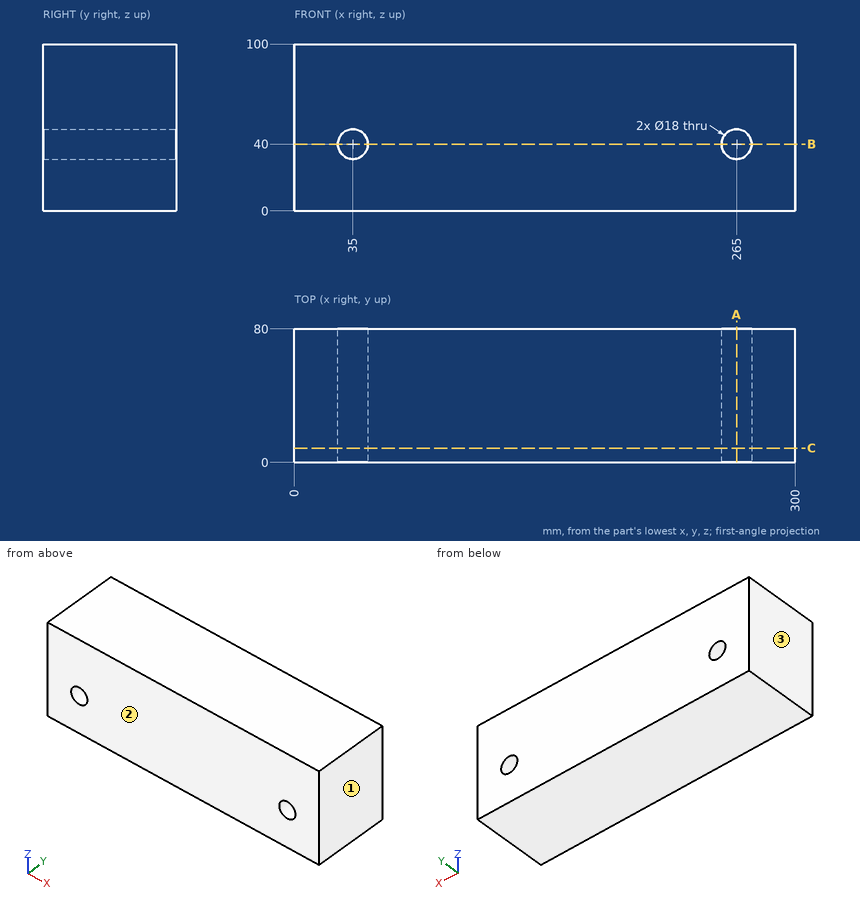
Source: three-view drawing plus pictorial views. Frame: mm from the lowest corner of the part. Coordinates: 2 decimals unless noted, no trailing zeros. Order: outer loops, then holes, each group sorted by start corner. A loop starts at its lowest first (then second) coordinate and runs counter-clockwise, first axis right, second up. Notation, with made-up numbers: M 65.25,71 L 101.25,71 A18 ccw 101.25,103 Z; hole C -40,49.25 d3. An arc over 180 degrees is marked long. One line per question, with ' | ' between items. Start each with the question number.
Item 1: Ray query, probe 1 along X at (y, z) = (58, 40); probe 2 along Z at (x, y) = (35, 35); probe 3 along X at (y, z) = (31.5, 35.5). Return the intervals inside material, ascending. Write a range as [from, to].
Item 2: Pin query (flat end, axial travel): pin 1 Ø11 at (x, z) = (35, 40) entering from +Y (1 decimal). Return the tip coordinate at first contact, or that it passes through.
Item 3: Cut plane B-B, the plane z = 40. Return the cut outline in (x, y).
Item 4: Cut plane A-A, the plane x = 265. Return the cut outline in (y, z).
Item 5: Draft query along X for the marked faces 1, 2 and 3. Return one class per face: released by +X, released by -X, zero draft, split by the parting line, or undercut.
Item 6: Cut plane C-C, the plane y = 8.5. Return the cut outline in (x, z).
A:
1) probe 1: x = [0, 26], [44, 256], [274, 300] | probe 2: z = [0, 31], [49, 100] | probe 3: x = [0, 27.21], [42.79, 257.21], [272.79, 300]
2) pin 1: passes through
3) outline: M 0,0 L 26,0 L 26,80 L 0,80 Z; M 44,0 L 256,0 L 256,80 L 44,80 Z; M 274,0 L 300,0 L 300,80 L 274,80 Z
4) outline: M 0,0 L 80,0 L 80,31 L 0,31 Z; M 0,49 L 80,49 L 80,100 L 0,100 Z
5) face 1: released by +X | face 2: zero draft | face 3: released by -X
6) outline: M 0,0 L 300,0 L 300,100 L 0,100 Z; hole C 35,40 d18; hole C 265,40 d18
